Check sheet for the modelled part. Datum: model origin and axes. Units: mm. Round coordinates to 2 decimals unless told otherwise and drop trailing zeros. Order: outer loops, then holes, each group sorted by start corner. A loop starts at its lowest first (then second) coordinate and runs counter-clockwise, first axis right, second up. Notation, with made-up numbers: (57, 53.5) -> (116, 53.5) arc R29 cw to (116, 74.5) -> close; hole circle Ø10 at (78.25, -37.75). An arc over 180 degrees is marked (long way). Answer in a Markdown table with one row per item. Add a question column.
1. Sectioned sample at A-A, the plane y = 0. Record the boundary of the cut face in (x, z), then the cut area to 3 significant figures.
2. Sectioned sample at B-B, the plane x = 61.5. Record the boundary of the cut face in (y, z).
3. Material ranges on L1, parallel to Z at x = 6.25, y = 0; L2, parallel to Y at x = 5.5, z = 0; L3, parallel to Z at x = 11, y = 1.5, recorded low to high. Write a range as from..to.
4. Depth check by flat-ended pin: P1, Ø4.5, axis at y = 0, z = -0.5, coming from the -X side; P2, Ø1.5, axis at x = 30, z = 1.5, coming from the +Y side; P3, Ø3, axis at x = 89.5, z = 3, coming from the +Y side. Enter the tip coordinate at first touch or a pass-through.
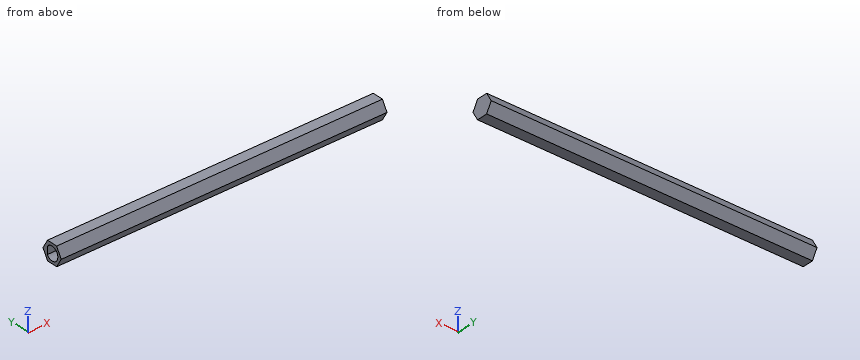
```python
from build123d import *

# Parameters (mm, degrees)
AXLE_DEPTH       = 142.24
DRIVE_SLOT_DEPTH = 13.97


with BuildPart() as part:
    # Hex Profile → Axle (new body)
    with BuildSketch(Plane(origin=(0, 0, 0), x_dir=(0, 0, -1), z_dir=(1, 0, 0))):
        Polygon((4.124445986, -2.38125), (4.124445986, 2.38125), (0, 4.7625), (-4.124445986, 2.38125), (-4.124445986, -2.38125), (0, -4.7625), align=None)
    extrude(amount=AXLE_DEPTH)

    # Motor Shaft Profile → Drive  Slot (cut)
    with BuildSketch(Plane.ZY):
        with BuildLine():
            Line((-1.669458355, 2.4892), (1.669458355, 2.4892))
            ThreePointArc((1.669458355, 2.4892), (0, -2.9972), (-1.669458355, 2.4892))
        make_face()
    extrude(amount=-DRIVE_SLOT_DEPTH, mode=Mode.SUBTRACT)


solid = part.part
```
Answer key:
| question | item | result |
|---|---|---|
| 1 | outline | (0, -4.12) -> (142.24, -4.12) -> (142.24, 4.12) -> (0, 4.12) -> (0, 3) -> (13.97, 3) -> (13.97, -3) -> (0, -3) -> close |
| 1 | area | 1,090 mm² |
| 2 | outline | (-4.76, 0) -> (-2.38, -4.12) -> (2.38, -4.12) -> (4.76, 0) -> (2.38, 4.12) -> (-2.38, 4.12) -> close |
| 3 | L1 | z = -4.12..-3, 3..4.12 |
| 3 | L2 | y = -4.76..-3, 2.49..4.76 |
| 3 | L3 | z = -4.12..-2.59, 2.59..4.12 |
| 4 | P1 | stops at x = 13.97 |
| 4 | P2 | stops at y = 4.33 |
| 4 | P3 | stops at y = 3.9 |
